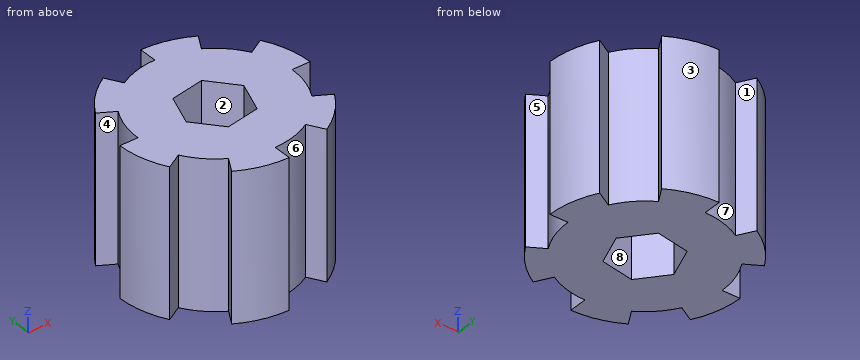
from build123d import *

# Parameters (mm, degrees)
DODANIE_WYCI_GNI_CIE1_DEPTH = 21.5


with BuildPart() as part:
    # Szkic1 → Dodanie-wyciągnięcie1 (new body)
    with BuildSketch(Plane.XY):
        with BuildLine():
            Line((0, 14), (0, 11.35))
            ThreePointArc((0, 11.35), (-2.937596162, 10.963258128), (-5.675, 9.829388333))
            Line((-5.675, 9.829388333), (-7, 12.124355653))
            ThreePointArc((-7, 12.124355653), (-9.899494937, 9.899494937), (-12.124355653, 7))
            Line((-12.124355653, 7), (-9.829388333, 5.675))
            ThreePointArc((-9.829388333, 5.675), (-10.963258128, 2.937596162), (-11.35, 0))
            Line((-11.35, 0), (-14, 0))
            ThreePointArc((-14, 0), (-13.522961568, -3.623466631), (-12.124355653, -7))
            Line((-12.124355653, -7), (-9.829388333, -5.675))
            ThreePointArc((-9.829388333, -5.675), (-8.025661966, -8.025661966), (-5.675, -9.829388333))
            Line((-5.675, -9.829388333), (-7, -12.124355653))
            ThreePointArc((-7, -12.124355653), (-3.623466631, -13.522961568), (0, -14))
            Line((0, -14), (0, -11.35))
            ThreePointArc((0, -11.35), (2.937596162, -10.963258128), (5.675, -9.829388333))
            Line((5.675, -9.829388333), (7, -12.124355653))
            ThreePointArc((7, -12.124355653), (9.899494937, -9.899494937), (12.124355653, -7))
            Line((12.124355653, -7), (9.829388333, -5.675))
            ThreePointArc((9.829388333, -5.675), (10.963258128, -2.937596162), (11.35, 0))
            Line((11.35, 0), (14, 0))
            ThreePointArc((14, 0), (13.522961568, 3.623466631), (12.124355653, 7))
            Line((12.124355653, 7), (9.829388333, 5.675))
            ThreePointArc((9.829388333, 5.675), (8.025661966, 8.025661966), (5.675, 9.829388333))
            Line((5.675, 9.829388333), (7, 12.124355653))
            ThreePointArc((7, 12.124355653), (3.623466631, 13.522961568), (0, 14))
        make_face()
        Polygon((4.922995461, 0.874137115), (1.704472782, 4.700507689), (-3.218522678, 3.826370574), (-4.922995461, -0.874137115), (-1.704472782, -4.700507689), (3.218522678, -3.826370574), align=None, mode=Mode.SUBTRACT)
    extrude(amount=DODANIE_WYCI_GNI_CIE1_DEPTH)


solid = part.part
Geometry: final body of the model. Coordinates: model frame, mm. Face numbers are marked on the shaded views. A direction names the side the tool comes from. Give positions to 0.01 mm unless a question says otherwise; leave off trailing zeros. Write each loop counter-clockwise with the first axis right and the second up, starting at its lowest first coordinate (ties: lowest second). Pieces come first, ordered by that corner, then holes. Notation, with made-up numbers: (-1, 42.5) -> (54, 42.5) arc R24 cw to (54, 74.5) -> close; hole circle Ø7 at (-29.5, 53.5). An arc over 180 degrees is marked (long way). Answer as a JSON object with one key per item and string values.
1. Cut plane C-C on x = -2.75. Output: boundary loops of the cut face in (y, z).
Ans:
{"outline": "(-13.73, 0) -> (-3.46, 0) -> (-3.46, 21.5) -> (-13.73, 21.5) -> close; (3.91, 0) -> (11.01, 0) -> (11.01, 21.5) -> (3.91, 21.5) -> close"}
2. Ray query, probe 1 along Y at (x, z) = (-0.25, 14.5); probe 2 along X at (y, z) = (-6.75, 6.5); probe 3 along Y at (x, z) = (2, 12.75). Return the intervals inside material, ascending. Write a range as from..to.
Ans:
{"probe 1": "y = -14..-4.44, 4.35..11.35", "probe 2": "x = -12.27..-11.69, -9.12..11.69", "probe 3": "y = -11.17..-4.04, 4.35..13.86"}
3. Contact query for flat-ended pins moving along their axis: pin 1 (3 mm diameter, centred on x = 12, z = 5.5, fed in from -Y); pin 2 (5 mm diameter, centred on x = 0.5, z = 14.5, fed in from -Y); pin 3 (1.3 mm diameter, centred on x = -13, z = 14.5, fed in from +Y); pin 4 (2 mm diameter, centred on y = 13, z = 14.5, fed in from -X). Output: stop coordinate, or through.
Ans:
{"pin 1": "stops at y = -9.26", "pin 2": "stops at y = -14", "pin 3": "stops at y = 0", "pin 4": "stops at x = -7.21"}
4. Access query for the marked faces 5, 6, 7 and 8. Directions: +Z, -Z, +X, -X, +Y, -Y. A direction counts if a zero-diameter tool reaches every point of the face in a straight line with its end or side. Return the directions, or none.
Ans:
{"face 5": "+Z, -Z, +X", "face 6": "+Z, -Z, -Y", "face 7": "+Z, -Z, +Y", "face 8": "+Z, -Z"}
5. Cut plane D-D on y = 8.75. Output: boundary loops of the cut face in (x, z).
Ans:
{"outline": "(-10.93, 0) -> (7.23, 0) -> (7.23, 21.5) -> (-10.93, 21.5) -> close"}
6. Mould query, pull axis X, two halves, no side actions, for the marked faces 1, 2, 3 and 4. Classes: pulls with the +X half, pulls with the -X half, needs draft (parallel to the pull), parting line crosses it, or undercut.
Ans:
{"face 1": "undercut", "face 2": "undercut", "face 3": "pulls with the +X half", "face 4": "pulls with the -X half"}
7. Cut plane A-A on y = 3. Output: boundary loops of the cut face in (x, z).
Ans:
{"outline": "(-10.95, 0) -> (-3.52, 0) -> (-3.52, 21.5) -> (-10.95, 21.5) -> close; (3.13, 0) -> (13.67, 0) -> (13.67, 21.5) -> (3.13, 21.5) -> close"}
